The listing builds one solid part. Answer for the finished solid, in the listing's coordinates (mm). Face numbers are marked on the shaded views. A direction names the side the tool comes from. Give positions to 0.01 mm unless a question says otherwise; leave off trailing zeros. Write each loop counter-clockwise with the first axis right and the second up, starting at its lowest first coordinate (ties: lowest second). Pieces come first, ordered by that corner, then holes. Notation, with made-up numbers: (-30, 71) -> (-5, 71) arc R20 cw to (-5, 104) -> close; hole circle Ø11 at (89, 49). An arc over 180 degrees is marked (long way). Use CSV: the item, a comma, the result in double quotes. Start each with the question number.
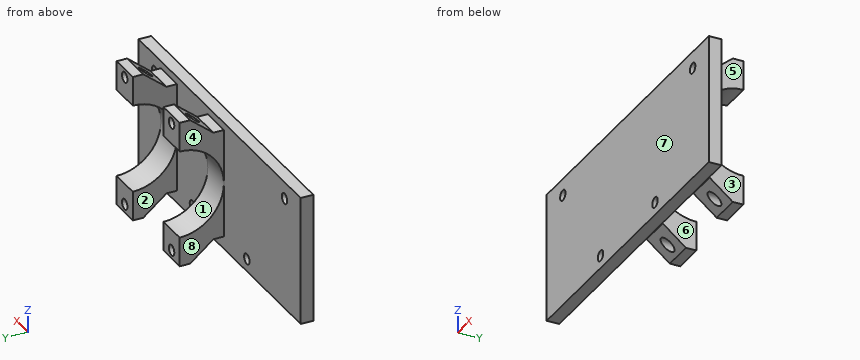
from build123d import *

# Parameters (mm, degrees)
CROQUIS1_W                = 149
CROQUIS1_H                = 53
SALIENTE_EXTRUIR1_DEPTH   = 6
SALIENTE_EXTRUIR2_DEPTH   = 15
SALIENTE_EXTRUIR5_DEPTH   = 15
CROQUIS3_R                = 21
CORTAR_EXTRUIR2_DEPTH     = 140.238105417
CROQUIS10_W               = 149
CROQUIS10_H               = 6
SALIENTE_EXTRUIR23_DEPTH  = 3
CROQUIS11_W               = 2.25
CROQUIS11_H               = 56
CORTAR_EXTRUIR3_DEPTH     = 93.895102131
CROQUIS12_W               = 56
CROQUIS12_H               = 6
SALIENTE_EXTRUIR24_DEPTH  = 3.75
CROQUIS13_W               = 150.5
CROQUIS13_H               = 0.5
CORTAR_EXTRUIR4_DEPTH     = 96.928684448
CROQUIS14_W               = 169.427236994
CROQUIS14_H               = 76.033419256
CORTAR_EXTRUIR5_DEPTH     = 88.876689173
SALIENTE_EXTRUIR25_DEPTH  = 15
CROQUIS16_R               = 2.5
CORTAR_EXTRUIR6_DEPTH     = 15
SIMETR_A2_COPY_1_DEPTH    = 15
SIMETR_A2_COPY_2_SKETCH_R = 2.5
SIMETR_A2_COPY_2_DEPTH    = 15
CROQUIS17_R               = 2.5
CORTAR_EXTRUIR7_DEPTH     = 89.255665541
CROQUIS19_W               = 150.5
CROQUIS19_H               = 6
SALIENTE_EXTRUIR26_DEPTH  = 6
CROQUIS20_R               = 2.5
CORTAR_EXTRUIR8_DEPTH     = 89.255665541


with BuildPart() as part:
    # Croquis1 → Saliente-Extruir1 (new body)
    with BuildSketch(Plane(origin=(0, 0, 0), x_dir=(1, 0, 0), z_dir=(0, 1, 0))):
        Rectangle(CROQUIS1_W, CROQUIS1_H)
    extrude(amount=SALIENTE_EXTRUIR1_DEPTH)

    # Croquis2 → Saliente-Extruir2 (add)
    with BuildSketch(Plane(origin=(51.5, 0, 0), x_dir=(0, 0, -1), z_dir=(1, 0, 0))):
        with BuildLine():
            Line((26, 6), (-26, 6))
            Line((-26, 6), (-26, 27))
            ThreePointArc((-26, 27), (0, 53), (26, 27))
            Line((26, 27), (26, 6))
        make_face()
    extrude(amount=-SALIENTE_EXTRUIR2_DEPTH)

    # Croquis5 → Saliente-Extruir5 (add)
    with BuildSketch(Plane.ZY.offset(-8)):
        with BuildLine():
            Line((-26, 6), (26, 6))
            Line((26, 6), (26, 27))
            ThreePointArc((26, 27), (0, 53), (-26, 27))
            Line((-26, 27), (-26, 6))
        make_face()
    extrude(amount=SALIENTE_EXTRUIR5_DEPTH)

    # Croquis3 → Cortar-Extruir2 (cut, through all)
    with BuildSketch(Plane(origin=(51.5, 0, 0), x_dir=(0, 0, -1), z_dir=(1, 0, 0))):
        with Locations(Location((0, 27, 0), (0, 0, 270))):
            Circle(CROQUIS3_R)
    extrude(amount=-CORTAR_EXTRUIR2_DEPTH, mode=Mode.SUBTRACT)

    # Croquis10 → Saliente-Extruir23 (add)
    with BuildSketch(Plane.XY.offset(26.5)):
        with Locations((0, 3)):
            Rectangle(CROQUIS10_W, CROQUIS10_H)
    extrude(amount=SALIENTE_EXTRUIR23_DEPTH)

    # Croquis11 → Cortar-Extruir3 (cut, through all)
    with BuildSketch(Plane(origin=(0, 6, 0), x_dir=(1, 0, 0), z_dir=(0, 1, 0))):
        with Locations((73.375, -1.5)):
            Rectangle(CROQUIS11_W, CROQUIS11_H)
    extrude(amount=-CORTAR_EXTRUIR3_DEPTH, mode=Mode.SUBTRACT)

    # Croquis12 → Saliente-Extruir24 (add)
    with BuildSketch(Plane.ZY.offset(74.5)):
        with Locations((1.5, 3)):
            Rectangle(CROQUIS12_W, CROQUIS12_H)
    extrude(amount=SALIENTE_EXTRUIR24_DEPTH)

    # Croquis13 → Cortar-Extruir4 (cut, through all)
    with BuildSketch(Plane(origin=(0, 6, 0), x_dir=(1, 0, 0), z_dir=(0, 1, 0))):
        with Locations((-3, 26.25)):
            Rectangle(CROQUIS13_W, CROQUIS13_H)
    extrude(amount=-CORTAR_EXTRUIR4_DEPTH, mode=Mode.SUBTRACT)

    # Croquis14 → Cortar-Extruir5 (cut, through all)
    with BuildSketch(Plane(origin=(0, 27, 0), x_dir=(-1, 0, 0), z_dir=(0, -1, 0))):
        Rectangle(CROQUIS14_W, CROQUIS14_H)
    extrude(amount=-CORTAR_EXTRUIR5_DEPTH, mode=Mode.SUBTRACT)

    # Croquis15 → Saliente-Extruir25 (add)
    with BuildSketch(Plane(origin=(51.5, 0, 0), x_dir=(0, 0, -1), z_dir=(1, 0, 0))):
        Polygon((-26, 27), (-35, 27), (-35, 22), (-26, 11), align=None)
    saliente_extruir25 = extrude(amount=-SALIENTE_EXTRUIR25_DEPTH)

    # Croquis16 → Cortar-Extruir6 (cut)
    with BuildSketch(Plane(origin=(0, 27, 0), x_dir=(1, 0, 0), z_dir=(0, 1, 0))):
        with Locations(Location((44, -31, 0), (0, 0, 270))):
            Circle(CROQUIS16_R)
    cortar_extruir6 = extrude(amount=-CORTAR_EXTRUIR6_DEPTH, mode=Mode.SUBTRACT)

    # Simetría1: Saliente-Extruir25, Cortar-Extruir6 across plane
    add(saliente_extruir25.mirror(Plane.ZY.offset(-22.25)))
    add(cortar_extruir6.mirror(Plane.ZY.offset(-22.25)), mode=Mode.SUBTRACT)

    # Simetría2: Saliente-Extruir25, Cortar-Extruir6 across plane
    add(saliente_extruir25.mirror(Plane.XY))
    add(cortar_extruir6.mirror(Plane.XY), mode=Mode.SUBTRACT)

    # Simetría2 copy 1 sketch → Simetría2 copy 1 (add)
    with BuildSketch(Plane.ZY.offset(7)):
        Polygon((-26, 27), (-35, 27), (-35, 22), (-26, 11), align=None)
    extrude(amount=-SIMETR_A2_COPY_1_DEPTH)

    # Simetría2 copy 2 sketch → Simetría2 copy 2 (cut)
    with BuildSketch(Plane(origin=(44.5, 27, 0), x_dir=(-1, 0, 0), z_dir=(0, 1, 0))):
        with Locations(Location((44, -31, 0), (0, 0, 270))):
            Circle(SIMETR_A2_COPY_2_SKETCH_R)
    extrude(amount=-SIMETR_A2_COPY_2_DEPTH, mode=Mode.SUBTRACT)

    # Croquis17 → Cortar-Extruir7 (cut, through all)
    with BuildSketch(Plane(origin=(0, 6, 0), x_dir=(1, 0, 0), z_dir=(0, 1, 0))):
        with Locations(Location((-63.25, -21.5, 0), (0, 0, 270))):
            Circle(CROQUIS17_R)
    cortar_extruir7 = extrude(amount=-CORTAR_EXTRUIR7_DEPTH, mode=Mode.SUBTRACT)

    # Croquis19 → Saliente-Extruir26 (add)
    with BuildSketch(Plane(origin=(0, 0, -26), x_dir=(-1, 0, 0), z_dir=(0, 0, -1))):
        with Locations((3, 3)):
            Rectangle(CROQUIS19_W, CROQUIS19_H)
    extrude(amount=SALIENTE_EXTRUIR26_DEPTH)

    # Simetría5: Cortar-Extruir7 across plane
    add(cortar_extruir7.mirror(Plane(origin=(-3, 0, 0), x_dir=(0, 0, 1), z_dir=(1, 0, 0))), mode=Mode.SUBTRACT)

    # Croquis20 → Cortar-Extruir8 (cut, through all)
    with BuildSketch(Plane(origin=(0, 6, 0), x_dir=(1, 0, 0), z_dir=(0, 1, 0))):
        with Locations(Location((22.25, 26, 0), (0, 0, 270))):
            Circle(CROQUIS20_R)
    cortar_extruir8 = extrude(amount=-CORTAR_EXTRUIR8_DEPTH, mode=Mode.SUBTRACT)

    # Simetría6: Cortar-Extruir8 across plane
    add(cortar_extruir8.mirror(Plane(origin=(-3, 0, 0), x_dir=(0, 0, 1), z_dir=(1, 0, 0))), mode=Mode.SUBTRACT)


solid = part.part
Q1. Section C-C on x = 0.5 is taken. Give the vertices of the cut face in (y, z), then the cut area to 3 significant figures.
Q2. Section B-B on x = -63.25 is taken. Give the vertices of the cut face in (y, z).
Q3. Flat-ended cylindrical pins translate along their axes: pin 1 Ø12 at (x, y) = (41.5, 7) entering from -Z; pin 2 Ø1 at (y, z) = (13.5, 22.5) entering from +X; pin 3 Ø5 at (x, y) = (14.5, 4) entering from +Z. Find the tip coordinate at first contact, or state that the pin passes through.
Q4. The mould has two halves that part along X. Classify the marked faces 5, 6, 7 and 8: +X half, -X half, draft (parallel to the pull), parting line (faces both ways), or undercut.
Q5. Straight lines are drawn through the part: L1, parallel to Z at x = 57.25, y = 1.8; L2, parallel to Z at x = -28.25, y = 3.1; L3, parallel to X at y = 9, z = -22. For each, find the intervals that lie inside material, in ascending order.
Q6. Section A-A on y = 24.5 is taken. Give the vertices of the cut face in (x, z).
Q7. For the marked faces 1, 2, 3 and 4, determine the directions among +Z, -Z, +X, -X, +Y, -Y from which every point of the face is accessible in a straight line to the end or side of a thin tool.
Q8. Section D-D on y = 8 is taken. Give the vertices of the cut face in (x, z).
Output:
1,outline,"(0, -32) -> (6, -32) -> (6, -26) -> (11, -26) -> (14.06, -28.5) -> (27, -28.5) -> (27, -21) arc R21 cw to (27, 21) -> (27, 28.5) -> (14.06, 28.5) -> (11, 26) -> (6, 26) -> (6, 29.5) -> (0, 29.5) -> close; (20.17, -33.5) -> (22, -35) -> (27, -35) -> (27, -33.5) -> close; (20.17, 33.5) -> (27, 33.5) -> (27, 35) -> (22, 35) -> close"
1,area,"858 mm²"
2,outline,"(0, -32) -> (6, -32) -> (6, 19) -> (0, 19) -> close; (0, 24) -> (6, 24) -> (6, 29.5) -> (0, 29.5) -> close"
3,pin 1,"z = -32"
3,pin 2,"x = 51.5"
3,pin 3,"z = 29.5"
4,face 5,"+X half"
4,face 6,"undercut"
4,face 7,"draft"
4,face 8,"-X half"
5,L1,"-32 to 19, 24 to 29.5"
5,L2,"-32 to -28.5, -23.5 to 29.5"
5,L3,"-7 to 8, 36.5 to 51.5"
6,outline,"(-7, -35) -> (8, -35) -> (8, -20.85) -> (-7, -20.85) -> close; (-7, 20.85) -> (8, 20.85) -> (8, 35) -> (-7, 35) -> close; (36.5, -35) -> (51.5, -35) -> (51.5, -20.85) -> (36.5, -20.85) -> close; (36.5, 20.85) -> (51.5, 20.85) -> (51.5, 35) -> (36.5, 35) -> close; hole circle Ø5 at (0.5, -31); hole circle Ø5 at (0.5, 31); hole circle Ø5 at (44, -31); hole circle Ø5 at (44, 31)"
7,face 1,"+X, -X, +Y"
7,face 2,"+Z, -Z, +Y"
7,face 3,"+Z, -Z, +X, +Y"
7,face 4,"+Z, -Z, -X, +Y"
8,outline,"(-7, -26) -> (8, -26) -> (8, -8.94) -> (-7, -8.94) -> close; (-7, 8.94) -> (8, 8.94) -> (8, 26) -> (-7, 26) -> close; (36.5, -26) -> (51.5, -26) -> (51.5, -8.94) -> (36.5, -8.94) -> close; (36.5, 8.94) -> (51.5, 8.94) -> (51.5, 26) -> (36.5, 26) -> close"
